For this review, take the finished solid that the model builds, in its own axes (mm). A direction names the side the tool comes from. Give positions to 0.01 mm unless a question says otherwise; leave off trailing zeros. Loops run counter-clockwise (first coordinate to the right, second up) from the corner with the lowest first, then second, coordinate; pieces in that order, holes last.
```python
from build123d import *

# Parameters (mm, degrees)
F1_DEPTH = 15


with BuildPart() as f1:
    # F0 (on Front) → F1 (new body, symmetric)
    with BuildSketch(Plane.XZ):
        Polygon((0, 0), (0, 30), (-80, 30), (-80, 230), (0, 230), (0, 260), (-110, 260), (-110, 0), align=None)
    extrude(amount=F1_DEPTH, both=True)

    # F2 (on Front) → F3 (revolve, cut)
    with BuildSketch(Plane.XZ):
        with BuildLine():
            Line((-20, 40), (-20, 20))
            ThreePointArc((-20, 20), (-10, 30), (-20, 40))
        make_face()
        with BuildLine():
            Line((-20, 240), (-20, 220))
            ThreePointArc((-20, 220), (-10, 230), (-20, 240))
        make_face()
    revolve(axis=Axis((-20, 0, 130), (0, 0, 1)), mode=Mode.SUBTRACT)


solid = f1.part
```
Item 1: Clearance check with flat-ended pins moving along their axes: pin 1 Ø5 at (y, z) = (-2, 63) entering from +X; pin 2 Ø2 at (x, z) = (-21, 227.5) entering from +Y. State where each tip first meets the part, or that it passes through.
Answer:
pin 1: stops at x = -80
pin 2: passes through
Item 2: For L1, parallel to Z at x = -52.5, y = 2.25; L2, parallel to X at y = 1.75, z = 210, list the stretches that pass through material, from the lowest coordinate up.
Answer:
L1: z = 0 to 30, 230 to 260
L2: x = -110 to -80
Item 3: Take a section at A-A on x = -63.5. Give the boundary of the cut face in (y, z), and give its area (3 significant figures).
Answer:
outline: (-15, 0) - (15, 0) - (15, 30) - (-15, 30) - close; (-15, 230) - (15, 230) - (15, 260) - (-15, 260) - close
area: 1,800 mm2
Item 4: Take a section at D-D on x = -17. Give the boundary of the cut face in (y, z).
Answer:
outline: (-15, 0) - (15, 0) - (15, 30) - (9.54, 30) arc R9.54 cw to (-9.54, 30) - (-15, 30) - close; (-15, 230) - (-9.54, 230) arc R9.54 cw to (9.54, 230) - (15, 230) - (15, 260) - (-15, 260) - close
Item 5: Tool access review of faces 1 (the flat face through (-39, 0, 30)), 2 (the flat face through (0, 0, 15)): name each direction out of +Z, -Z, +X, -X, +Y, -Y from which nothing blocks a thin tool from reaching the whole face with its end or side.
Answer:
face 1: +X, +Y, -Y
face 2: +Z, -Z, +X, +Y, -Y
Item 6: Take a section at B-B on z = 98. Give the boundary of the cut face in (x, y), and give its area (3 significant figures).
Answer:
outline: (-110, -15) - (-80, -15) - (-80, 15) - (-110, 15) - close
area: 900 mm2
Item 7: Take a section at C-C on y = -6.75. Give the boundary of the cut face in (x, z), and give its area (3 significant figures).
Answer:
outline: (-110, 0) - (0, 0) - (0, 30) - (-12.62, 30) arc R7.38 cw to (-27.38, 30) - (-80, 30) - (-80, 230) - (-27.38, 230) arc R7.38 cw to (-12.62, 230) - (0, 230) - (0, 260) - (-110, 260) - close
area: 12,400 mm2
Item 8: The part is to be moulded in two halves that separate along Z. For faces 3 (the flat face through (-80.2, 15, 131.8)), 4 (the flat face through (-56, 0, 0)), 5 (the flat face through (-41, 0, 230)), 6 (the flat face through (-54, 0, 260)), say which applies: released by +Z, released by -Z, zero draft, split by the parting line, or undercut.
Answer:
face 3: zero draft
face 4: released by -Z
face 5: undercut
face 6: released by +Z
